Input: part model. Units: mm. Frame: model coordinates. A direction names the side the tool comes from. Coordinates: 2 decimals unless noted, no trailing zeros. Write each loop counter-clockwise with the first axis right and the second up, starting at its lowest first coordinate (ties: lowest second). Pieces come first, ordered by that corner, then holes.
1) Section query B-B (y = 10.5). Output: boundary loops of the cut face in (x, z), then the cut area to 3 significant figures.
2) Set-up query: faces 1 (the flat face through (-6, 16.6, 4.6)), 2 (the flat face through (-0.1, 12.4, 4.6)), 3 (the cylindrical face through (-3.7, 0.43, 0.4)). Return all of +Z, -Z, +X, -X, +Y, -Y with unobstructed straight access to the full face (end or side cutting, diameter ignored); none if empty.
3) Draft query along X for faces 4 (the cylindrical face through (-3.68, 7.58, -4.55)), 5 (the flat face through (6, 16.6, 4.6)), 6 (the conical face through (-2.209, 17.237, 4.506)). Return one class per face: pulls with the +X half, pulls with the -X half, needs draft (parallel to the pull), parting line crosses it, or undercut.
4) Line query: L1, parallel to X at y = 9.5, z = 4; L2, parallel to Y at x = 7, z = 0; L3, parallel to Y at x = 4.75, z = 3. Output: solid intervals per line, ascending.
5) Pin query (flat end, axial travel): pin 1 Ø12 at (x, y) = (1, 23.5) entering from -Z; pin 2 Ø1.4 at (y, z) = (28, 3.5) entering from -X; pin 3 Ø2 at (x, z) = (-0.5, 0.5) entering from -Y. Return the tip coordinate at first contact, or that it passes through.
6) Section query C-C (x = 7.75). Output: boundary loops of the cut face in (y, z), then the cut area to 3 significant figures.
7) Section query D-D (y = 38). Output: boundary loops of the cut face in (x, z).
8) Section query A-A (y = 5). Output: boundary loops of the cut face in (x, z), then the cut area to 3 significant figures.
from build123d import *

# Parameters (mm, degrees)
SKETCH1_W           = 20
SKETCH1_H           = 10
BOSS_EXTRUDE1_DEPTH = 10
SKETCH2_R           = 2.15
CUT_EXTRUDE1_DEPTH  = 23.912878475
SKETCH3_W           = 4
SKETCH3_H           = 4
BOSS_EXTRUDE2_DEPTH = 35
BOSS_EXTRUDE3_REACH = 51.497
SKETCH4_W           = 10
SKETCH4_H           = 7
SKETCH5_W           = 6.5
SKETCH5_H           = 10
CUT_EXTRUDE2_DEPTH  = 12
FILLET1_R           = 1.5
CHAMFER1_SIZE       = 0.8


with BuildPart() as part:
    # Sketch1 → Boss-Extrude1 (new body)
    with BuildSketch(Plane(origin=(0, 0, 0), x_dir=(1, 0, 0), z_dir=(0, 1, 0))):
        Rectangle(SKETCH1_W, SKETCH1_H)
    extrude(amount=BOSS_EXTRUDE1_DEPTH)

    # Sketch2 → Cut-Extrude1 (cut, through all)
    with BuildSketch(Plane(origin=(10, 0, 0), x_dir=(0, 0, -1), z_dir=(1, 0, 0))):
        with Locations((0, 5)):
            Circle(SKETCH2_R)
    extrude(amount=-CUT_EXTRUDE1_DEPTH, mode=Mode.SUBTRACT)

    # Sketch3 → Boss-Extrude2 (add)
    with BuildSketch(Plane(origin=(0, 10, 0), x_dir=(1, 0, 0), z_dir=(0, 1, 0))):
        with Locations((0, -3)):
            Rectangle(SKETCH3_W, SKETCH3_H)
    extrude(amount=BOSS_EXTRUDE2_DEPTH)

    # Boss-Extrude3: up to this face of the body (flat: up to its plane)
    boss_extrude3_end = Plane(part.part.faces().sort_by_distance((-10, 5, -4.858578644))[0])
    # Sketch4 → Boss-Extrude3 (add, up to the picked face)
    with BuildSketch(Plane(origin=(10, 0, 0), x_dir=(0, 0, -1), z_dir=(1, 0, 0)), mode=Mode.PRIVATE) as boss_extrude3_sk1:
        with Locations((0, 13.5)):
            Rectangle(SKETCH4_W, SKETCH4_H)
    boss_extrude3_tool1 = split(extrude(boss_extrude3_sk1.sketch, amount=-BOSS_EXTRUDE3_REACH, mode=Mode.PRIVATE), bisect_by=boss_extrude3_end, keep=Keep.BOTH, mode=Mode.PRIVATE)
    add(boss_extrude3_tool1.solids().sort_by(Axis((10, 13.5, 0), (-1, 0, 0)))[0])

    # Sketch5 → Cut-Extrude2 (cut)
    with BuildSketch(Plane.XZ):
        Rectangle(SKETCH5_W, SKETCH5_H)
    extrude(amount=-CUT_EXTRUDE2_DEPTH, mode=Mode.SUBTRACT)

    # Fillet1
    fillet1_edges = [part.edges().sort_by_distance(p)[0] for p in [
        (-2, 31, 1),
        (2, 31, 1),
        (-2, 45, 3),
        (2, 45, 3),
        (0, 45, 1),
        (0, 17, 1),
        (-2, 17, 3),
        (2, 17, 3),
        (0, 17, -5),
        (10, 17, 0),
        (-10, 17, 0),
        (-10, 0, 0),
        (-6.625, 0, -5),
        (6.625, 0, -5),
        (-3.25, 6, -5),
        (10, 0, 0),
        (0, 12, -5),
        (3.25, 6, -5),
        (-3.25, 0, 0),
        (3.25, 0, 0),
        (-10, 8.5, -5),
        (10, 8.5, -5),
    ]]
    fillet(fillet1_edges, radius=FILLET1_R)

    # Chamfer1
    chamfer1_edges = [part.edges().sort_by_distance(p)[0] for p in [
        (-6.625, 0, 5),
        (-9.560660172, 16.560660172, 5),
        (9.560660172, 16.560660172, 5),
        (-9.560660172, 0.439339828, 5),
        (9.560660172, 0.439339828, 5),
        (3.689339828, 0.439339828, 5),
        (-3.689339828, 0.439339828, 5),
        (-1.560660172, 44.560660172, 5),
        (1.560660172, 44.560660172, 5),
        (-2.439339828, 17.439339828, 5),
        (2.439339828, 17.439339828, 5),
        (3.25, 6.75, 5),
        (0, 12, 5),
        (-3.25, 6.75, 5),
        (-2, 31, 5),
        (6, 17, 5),
        (-6, 17, 5),
        (2, 31, 5),
        (0, 45, 5),
        (6.625, 0, 5),
        (10, 8.5, 5),
        (-10, 8.5, 5),
    ]]
    chamfer(chamfer1_edges, length=CHAMFER1_SIZE)


solid = part.part
Answer:
1. outline: (-10, -3.5) arc R1.5 ccw to (-8.5, -5) - (-4.75, -5) arc R1.5 ccw to (-3.25, -3.5) - (-3.25, 4.2) - (-4.05, 5) - (-9.2, 5) - (-10, 4.2) - close; (3.25, -3.5) arc R1.5 ccw to (4.75, -5) - (8.5, -5) arc R1.5 ccw to (10, -3.5) - (10, 4.2) - (9.2, 5) - (4.05, 5) - (3.25, 4.2) - close
1. area: 132 mm2
2. face 1: +Z, -X, +Y
2. face 2: +Z, -Y
2. face 3: +Z, -Z, -Y
3. face 4: undercut
3. face 5: needs draft
3. face 6: pulls with the -X half
4. L1: x = -10 to -3.25, 3.25 to 10
4. L2: y = 0 to 2.85, 7.15 to 17
4. L3: y = 0 to 17
5. pin 1: stops at z = 0.63
5. pin 2: stops at x = -2
5. pin 3: stops at y = 12
6. outline: (0, -3.5) arc R1.5 ccw to (1.5, -5) - (15.5, -5) arc R1.5 ccw to (17, -3.5) - (17, 4.2) - (16.2, 5) - (0.8, 5) - (0, 4.2) - close; hole circle Ø4.3 at (5, 0)
6. area: 154 mm2
7. outline: (-2, 2.5) arc R1.5 ccw to (-0.5, 1) - (0.5, 1) arc R1.5 ccw to (2, 2.5) - (2, 4.2) - (1.2, 5) - (-1.2, 5) - (-2, 4.2) - close
8. outline: (-10, -3.5) arc R1.5 ccw to (-8.5, -5) - (-4.75, -5) arc R1.5 ccw to (-3.25, -3.5) - (-3.25, -2.15) - (-10, -2.15) - close; (-10, 2.15) - (-3.25, 2.15) - (-3.25, 4.2) - (-4.05, 5) - (-9.2, 5) - (-10, 4.2) - close; (3.25, -3.5) arc R1.5 ccw to (4.75, -5) - (8.5, -5) arc R1.5 ccw to (10, -3.5) - (10, -2.15) - (3.25, -2.15) - close; (3.25, 2.15) - (10, 2.15) - (10, 4.2) - (9.2, 5) - (4.05, 5) - (3.25, 4.2) - close
8. area: 73.7 mm2
